```python
from build123d import *

# Parameters (mm, degrees)
IZIM1_W                     = 14.5
IZIM1_H                     = 26
IZIM1_W_2                   = 12.5
IZIM1_H_2                   = 24
Y_KSEKLIK_EKSTR_ZYON1_DEPTH = 15
IZIM2_W                     = 14.5
IZIM2_H                     = 26
Y_KSEKLIK_EKSTR_ZYON2_DEPTH = 1
KES_EKSTR_ZYON1_DEPTH       = 2


with BuildPart() as part:
    # Çizim1 → Yükseklik-Ekstrüzyon1 (new body)
    with BuildSketch(Plane(origin=(0, 0, 0), x_dir=(1, 0, 0), z_dir=(0, 1, 0))):
        Rectangle(IZIM1_W, IZIM1_H)
        Rectangle(IZIM1_W_2, IZIM1_H_2, mode=Mode.SUBTRACT)
    extrude(amount=Y_KSEKLIK_EKSTR_ZYON1_DEPTH)

    # Çizim2 → Yükseklik-Ekstrüzyon2 (add)
    with BuildSketch(Plane(origin=(0, 15, 0), x_dir=(1, 0, 0), z_dir=(0, 1, 0))):
        Rectangle(IZIM2_W, IZIM2_H)
    extrude(amount=Y_KSEKLIK_EKSTR_ZYON2_DEPTH)

    # Çizim3 → Kes-Ekstrüzyon1 (cut)
    with BuildSketch(Plane.XY.offset(13)):
        Polygon((4.5, 11), (0, 11), (-4.5, 11), (-4.5, 7.5), (4.5, 7.5), align=None)
    extrude(amount=-KES_EKSTR_ZYON1_DEPTH, mode=Mode.SUBTRACT)


solid = part.part
```
Check sheet for the modelled part. Datum: model origin and axes. Units: mm. A direction names the side the tool comes from. Coordinates: 2 decimals unless noted, no trailing zeros. Order: outer loops, then holes, each group sorted by start corner. A loop starts at its lowest first (then second) coordinate and runs counter-clockwise, first axis right, second up. Notation, with made-up numbers: (23, -28.75) -> (77, -28.75) arc R25 cw to (77, 4.25) -> close; hole circle Ø6 at (61.5, 50.5). An arc over 180 degrees is marked (long way). Write item = value, one per line. Start each with the question number.
1) Access from +Z, -Z, +X, -X, +Y, -Y to the whole of each face (thin tool, end or side, straight path). Record for faces 1 (the flat face through (0, 16, 0)), 2 (the flat face through (-0.1, 7.5, 12.5)), 3 (the flat face through (-6.25, 7, 0)).
2) Cross-section at B-B (z = 4). Enter the section's corners in (x, y).
3) Mould release check, pull along Z, two halves, no side actions. Record for faces 4 (the flat face through (0, 6, 13)), 5 (the flat face through (0, 15, 0)), 6 (the flat face through (4.5, 9.2, 12.5)), 7 (the flat face through (0, 7, -12)): +Z half, -Z half, draft (parallel to the pull), parting line (faces both ways), or undercut.
4) Cross-section at A-A (x = -2). Enter the section's corners in (y, z).
5) Cross-section at D-D (x = 5). Enter the section's corners in (y, z).
6) Cross-section at C-C (y = 6.5). Enter the section's corners in (x, z), then the cut area to 3 significant figures.
7) Material ranges on L1, parallel to X at y = 1.5, z = -4; L2, parallel to Z at x = 3.5, y = 2; L3, parallel to Z at x = -1.5, y = 7.75, recorded low to high.
Ans:
q1.face_1 = +Z, -Z, +X, -X, +Y
q1.face_2 = +Z
q1.face_3 = -Y
q2.outline = (-7.25, 0) -> (-6.25, 0) -> (-6.25, 15) -> (6.25, 15) -> (6.25, 0) -> (7.25, 0) -> (7.25, 16) -> (-7.25, 16) -> close
q3.face_4 = +Z half
q3.face_5 = undercut
q3.face_6 = draft
q3.face_7 = undercut
q4.outline = (0, -13) -> (16, -13) -> (16, 13) -> (11, 13) -> (11, 12) -> (15, 12) -> (15, -12) -> (0, -12) -> close; (0, 12) -> (7.5, 12) -> (7.5, 13) -> (0, 13) -> close
q5.outline = (0, -13) -> (16, -13) -> (16, 13) -> (0, 13) -> (0, 12) -> (15, 12) -> (15, -12) -> (0, -12) -> close
q6.outline = (-7.25, -13) -> (7.25, -13) -> (7.25, 13) -> (-7.25, 13) -> close; hole (-6.25, -12) -> (6.25, -12) -> (6.25, 12) -> (-6.25, 12) -> close
q6.area = 77.0 mm²
q7.L1 = -7.25 to -6.25, 6.25 to 7.25
q7.L2 = -13 to -12, 12 to 13
q7.L3 = -13 to -12
